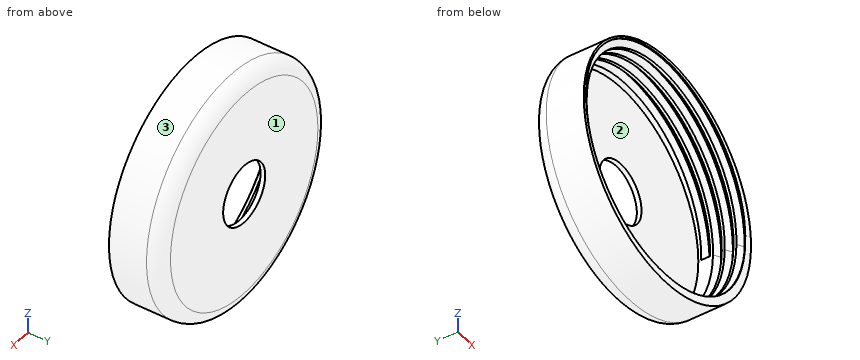
from build123d import *

# Parameters (mm, degrees)
SKETCH1_W     = 17.15
SKETCH1_H     = 1
THREAD1_PITCH = 2.5
FILLET1_R     = 3


with BuildPart() as part:
    # Sketch1 → Revolve1 (revolve)
    with BuildSketch(Plane.XY, mode=Mode.PRIVATE) as revolve1_sk:
        with Locations((14.925, 10.5)):
            Rectangle(SKETCH1_W, SKETCH1_H)
        Polygon((23.5, 11), (23.5, 10), (23.5, 0), (25.25, 0), (25.25, 11), align=None)
    revolve(revolve1_sk.sketch.rotate(Axis((0, 10, 0), (0, -1, 0)), 180), axis=Axis((0, 10, 0), (0, -1, 0)))

    # Thread1: the profile of Thread Profile1 profile screwed along a right-hand helix of 4 turns, 10 arcs to a turn; built about Z, then put on its axis
    thread1_z = Axis((0, 0, 0), (0, 0, 1))
    thread1_corners = [(23.4997, 0, -0.000173205), (24.853164688, 0, 0.781249997), (24.853164688, 0, 1.093749997), (23.4997, 0, 1.875173198)]
    with BuildLine(mode=Mode.PRIVATE) as thread1_profile:
        Line(thread1_corners[0], thread1_corners[1])
        Line(thread1_corners[1], thread1_corners[2])
        Line(thread1_corners[2], thread1_corners[3])
        Line(thread1_corners[3], thread1_corners[0])
    thread1_cap = Face(thread1_profile.wire())
    thread1_turn_angles = [0, 18, 36, 54, 72, 90, 108, 126, 144, 162, 180, 198, 216, 234, 252, 270, 288, 306, 324, 342, 360]
    thread1_turn_weights = [1, 0.9510565162951535, 1, 0.9510565162951535, 1, 0.9510565162951535, 1, 0.9510565162951535, 1, 0.9510565162951535, 1, 0.9510565162951535, 1, 0.9510565162951535, 1, 0.9510565162951535, 1, 0.9510565162951535, 1, 0.9510565162951535, 1]
    thread1_turn_rails = [Edge.make_bspline([Vector(p[0], p[1], 0).rotate(thread1_z, thread1_turn_angles[k]) / thread1_turn_weights[k] + Vector(0, 0, p[2] + THREAD1_PITCH * thread1_turn_angles[k] / 360) for k in range(21)], [0, 0, 0, 1, 1, 2, 2, 3, 3, 4, 4, 5, 5, 6, 6, 7, 7, 8, 8, 9, 9, 10, 10, 10], 2, thread1_turn_weights) for p in thread1_corners]
    thread1_turn_sides = [Face.make_surface_from_curves(thread1_turn_rails[p[0]], thread1_turn_rails[p[1]]) for p in [(0, 1), (1, 2), (2, 3), (3, 0)]]
    thread1 = Plane(origin=(0, -2.5, 0), x_dir=(1, 0, 0), z_dir=(0, 1, 0)) * Solid(Shell([*[p.moved(Location((0, 0, THREAD1_PITCH * i))) for i in range(4) for p in thread1_turn_sides], thread1_cap, thread1_cap.rotate(thread1_z, 1440).moved(Location((0, 0, THREAD1_PITCH * 1440 / 360)))]))
    add(thread1, mode=Mode.SUBTRACT)

    # Fillet1
    fillet1_edges = [part.edges().sort_by_distance(p)[0] for p in [
        (25.25, 11, 0),
    ]]
    fillet(fillet1_edges, radius=FILLET1_R)


solid = part.part
The listing builds one solid part. Answer for the finished solid, in the listing's coordinates (mm). Face numbers are marked on the shaded views. Give positions to 0.01 mm unless a question says otherwise; leave off trailing zeros. One line per question, with ' | ' between items. Start each with the question number.
1. Find the intervals of material crossed by probe 1 along Y at (x, z) = (-9.5, 1); probe 2 along Z at (x, y) = (8, 5.75); probe 3 along Z at (x, y) = (-3.5, 7.5), in increasing order.
2. Given pin 1 Ø1.5 at (y, z) = (6.5, 10) entering from -X; pin 2 Ø1.5 at (x, z) = (-15.5, 15) entering from -Y; pin 3 Ø3 at (x, y) = (9, 5.5) entering from -Z, each flat-ended and moving along its own axis, determine where each tip first touches the part or whether it passes through.
3. For a pull along Z with two mould halves and no side action, classify the marked faces 1, 2 and 3 as pulls with the +Z half, pulls with the -Z half, needs draft (parallel to the pull), parting line crosses it, or undercut.
Response values:
1) probe 1: 10 to 11 | probe 2: -23.95 to -22.58, 23.26 to 23.95 | probe 3: -25.01 to -23.34, 24.43 to 25.01
2) pin 1: x = -23.49 | pin 2: y = 10 | pin 3: z = -24.11
3) face 1: needs draft | face 2: undercut | face 3: parting line crosses it
